Could you check a few things on this model? Use its own coordinates, in mm. Face numbers are marked on the shaded views. A direction names the side the tool comes from. Round coordinates to 2 decimals unless told otherwise and drop trailing zeros. Order: outer loops, then holes, each group sorted by start corner. A loop starts at its lowest first (then second) coordinate and runs counter-clockwise, first axis right, second up. Notation, with made-up numbers: M -7,12.5 L 19,12.5 A7 ccw 19,17.5 Z; hole C 83,-3.75 d6. An arc over 180 degrees is marked long. Write each question's results on one line, items separated by ' | '. Start each with the question number.
1. Suppose I cut it at B-B on x = -37.5. Write out the boundary of the cut face in (y, z).
2. We'd pull the mould along Z, two halves only. Please class the marked faces 3, 4, 5 and 6: released by +Z, released by -Z, zero draft, split by the parting line, or undercut.
3. Please list where these lines run through material, in increasing order: L1, parallel to Z at x = -35, y = -20; L2, parallel to Y at x = -42.5, z = -39.5; L3, parallel to Z at x = -31, y = -20.5.
4. Suppose I cut it at A-A on y = -20.5. Write out the boundary of the cut face in (x, z).
5. I'm going to push a flat-ended pin straight in: pin 1 (12.5 mm diameter, centred on y = -18, z = -5, fed in from -X). Where does the tip first touch, or does it pass through?
6. Suppose I cut it at C-C on z = -38. Write out the boundary of the cut face in (x, y), and give its area (3 significant figures).
7. For the marked faces 1 and 2, which set-ups out of +Z, -Z, +X, -X, +Y, -Y let a thin tool reach every point of the face, with its end or its side?
8. Suppose I cut it at D-D on y = -38. Write out the boundary of the cut face in (x, z), and give its area (3 significant figures).
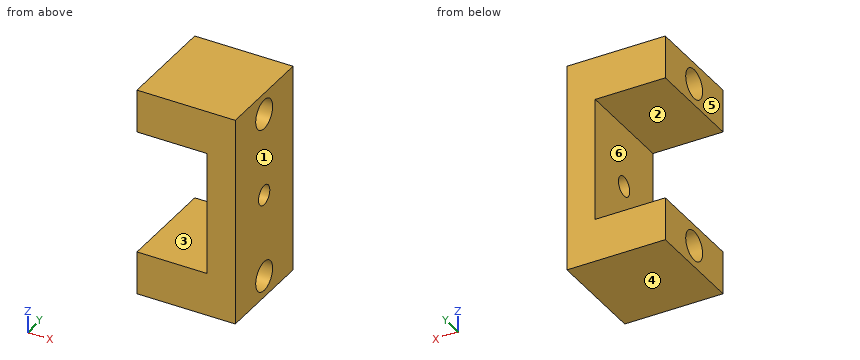
from build123d import *

# Parameters (mm, degrees)
F1_DEPTH = 41
F3_D     = 12
F5_D     = 12
F7_D     = 8


with BuildPart() as f1:
    # F0 (on Front) → F1 (new body)
    with BuildSketch(Plane.XZ):
        Polygon((-22.088847, 37.038844), (-62.088847, 37.038844), (-62.088847, 19.538844), (-33.588847, 19.538844), (-33.588847, -30.661156), (-62.088847, -30.661156), (-62.088847, -48.161156), (-22.088847, -48.161156), align=None)
    extrude(amount=F1_DEPTH)

    # F3 (through all)
    with Locations(Plane(origin=(-62.088847, 0, 0), x_dir=(0, -1, 0), z_dir=(-1, 0, 0))):
        with Locations((20.5, 28.288844)):
            Hole(F3_D / 2)

    # F5 (through all)
    with Locations(Plane(origin=(-62.088847, 0, 0), x_dir=(0, -1, 0), z_dir=(-1, 0, 0))):
        with Locations((20.5, -39.411156)):
            Hole(F5_D / 2)

    # F7 (through all)
    with Locations(Plane.YZ.offset(-22.088847)):
        with Locations((-20.5, -5.561156)):
            Hole(F7_D / 2)


solid = f1.part
Filled sheet:
1) outline: M -41,-48.16 L 0,-48.16 L 0,-30.66 L -41,-30.66 Z; M -41,19.54 L 0,19.54 L 0,37.04 L -41,37.04 Z; hole C -20.5,-39.41 d12; hole C -20.5,28.29 d12
2) face 3: undercut | face 4: released by -Z | face 5: zero draft | face 6: undercut
3) L1: z = -48.16 to -45.39, -33.43 to -30.66, 19.54 to 22.31, 34.27 to 37.04 | L2: y = -41 to -26.5, -14.5 to 0 | L3: z = -48.16 to -45.41, -33.41 to -9.56, -1.56 to 22.29, 34.29 to 37.04
4) outline: M -62.09,-48.16 L -22.09,-48.16 L -22.09,-45.41 L -62.09,-45.41 Z; M -62.09,-33.41 L -22.09,-33.41 L -22.09,-9.56 L -33.59,-9.56 L -33.59,-30.66 L -62.09,-30.66 Z; M -62.09,19.54 L -33.59,19.54 L -33.59,-1.56 L -22.09,-1.56 L -22.09,22.29 L -62.09,22.29 Z; M -62.09,34.29 L -22.09,34.29 L -22.09,37.04 L -62.09,37.04 Z
5) pin 1: stops at x = -33.59
6) outline: M -62.09,-41 L -22.09,-41 L -22.09,-26.33 L -62.09,-26.33 Z; M -62.09,-14.67 L -22.09,-14.67 L -22.09,0 L -62.09,0 Z | area: 1,170 mm^2
7) face 1: +Z, -Z, +X, +Y, -Y | face 2: -X, +Y, -Y
8) outline: M -62.09,-48.16 L -22.09,-48.16 L -22.09,37.04 L -62.09,37.04 L -62.09,19.54 L -33.59,19.54 L -33.59,-30.66 L -62.09,-30.66 Z | area: 1,980 mm^2
